Verification items for the finished model (mm, model axes). Face numbers are marked on the shaded views. Coordinates: 2 decimals unless noted, no trailing zeros. Order: outer loops, then holes, each group sorted by start corner. A loop starts at its lowest first (then second) coordinate and runs counter-clockwise, first axis right, second up. Notation, with made-up numbers: M 52.5,14 L 110.5,14 A30 ccw 110.5,45 Z; hole C -34,40 d10. An arc over 180 degrees is marked long. Return JSON: item names as keys, results as strings. Group by question number.
1. Mould release check, pull along X, two halves, no side actions. Record for the marked faces 1, 2 and 3: +X half, -X half, draft (parallel to the pull), parting line (faces both ways), or undercut.
2. Gauge pin test, flat ends, axial feed: pin 1 (1.5 mm diameter, centred on x = 1, z = 1, fed in from +Y); pin 2 (1.5 mm diameter, centred on y = 2, z = 10, fed in from -X); pin 3 (14.5 mm diameter, centred on x = 0, z = 0, fed in from +Y). Record the tip position at first contact, or that the pin passes through.
3. Section check C-C, the plane y = 6.5. Record the cut outline in (x, z).
4. Section check B-B, the plane z = 0. Record the cut outline in (x, y), plus the area to 3 significant figures.
5. Section check A-A, the plane x = 0. Record the cut outline in (y, z).
6. Section check D-D, the plane x = 3. Record the cut outline in (y, z), plus the area to 3 significant figures.
7. Material ranges on line 1 along Y through (x, z) = (2, 6.25); line 2 along X through (y, z) = (1.75, 0); line 3 along Z through (x, y) = (5.25, 7), recorded low to high.
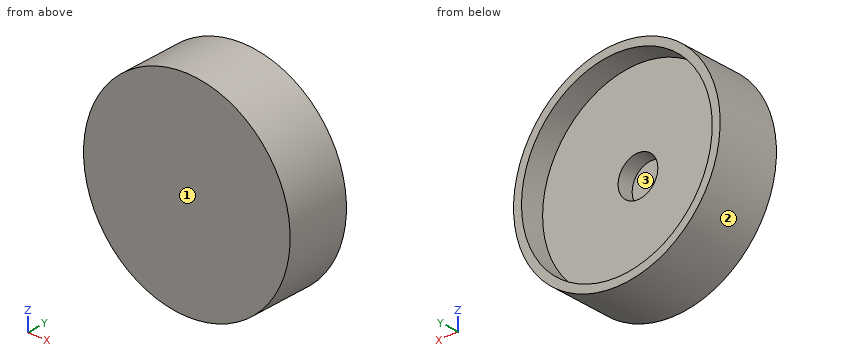
```python
from build123d import *

# Parameters (mm, degrees)
SKETCH_1_R          = 13
EXTRUDE_1_DEPTH     = 8
SKETCH_2_R          = 12
CUT_EXTRUDE_1_DEPTH = 3
SKETCH_3_R          = 2.5
CUT_EXTRUDE_2_DEPTH = 2


with BuildPart() as part:
    # 草图1 → 凸台-拉伸1 (new body)
    with BuildSketch(Plane(origin=(0, 0, 0), x_dir=(1, 0, 0), z_dir=(0, 1, 0))):
        with Locations(Location((0, 0, 0), (0, 0, 270))):
            Circle(SKETCH_1_R)
    extrude(amount=EXTRUDE_1_DEPTH)

    # 草图2 → 切除-拉伸1 (cut)
    with BuildSketch(Plane(origin=(0, 8, 0), x_dir=(1, 0, 0), z_dir=(0, 1, 0))):
        with Locations(Location((0, 0, 0), (0, 0, 270))):
            Circle(SKETCH_2_R)
    extrude(amount=-CUT_EXTRUDE_1_DEPTH, mode=Mode.SUBTRACT)

    # 草图3 → 切除-拉伸2 (cut)
    with BuildSketch(Plane(origin=(0, 5, 0), x_dir=(1, 0, 0), z_dir=(0, 1, 0))):
        with Locations(Location((0, 0, 0), (0, 0, 270))):
            Circle(SKETCH_3_R)
    extrude(amount=-CUT_EXTRUDE_2_DEPTH, mode=Mode.SUBTRACT)


solid = part.part
```
Answers follow:
{
 "1": {"face 1": "draft", "face 2": "parting line", "face 3": "undercut"},
 "2": {"pin 1": "y = 3", "pin 2": "x = -9.13", "pin 3": "y = 5"},
 "3": {"outline": "C 0,0 d26; hole C 0,0 d24"},
 "4": {"outline": "M -13,0 L 13,0 L 13,8 L 12,8 L 12,5 L 2.5,5 L 2.5,3 L -2.5,3 L -2.5,5 L -12,5 L -12,8 L -13,8 Z", "area": "126 mm^2"},
 "5": {"outline": "M 0,-13 L 8,-13 L 8,-12 L 5,-12 L 5,-2.5 L 3,-2.5 L 3,2.5 L 5,2.5 L 5,12 L 8,12 L 8,13 L 0,13 Z"},
 "6": {"outline": "M 0,-12.65 L 8,-12.65 L 8,-11.62 L 5,-11.62 L 5,11.62 L 8,11.62 L 8,12.65 L 0,12.65 Z", "area": "133 mm^2"},
 "7": {"line 1": "0 to 5", "line 2": "-13 to 13", "line 3": "-11.89 to -10.79, 10.79 to 11.89"}
}
